from build123d import *

# Parameters (mm, degrees)
SKETCH1_W           = 70
SKETCH1_H           = 160
BOSS_EXTRUDE1_DEPTH = 6.35
SKETCH7_W           = 4.699
SKETCH7_H           = 2.5
FILLET1_R           = 18
SKETCH11_R          = 1.65
CUT_EXTRUDE4_DEPTH  = 3.5
SKETCH14_R          = 1.25
CUT_EXTRUDE7_DEPTH  = 3.5


with BuildPart() as part:
    # Sketch1 → Boss-Extrude1 (new body)
    with BuildSketch(Plane(origin=(0, 0, 0), x_dir=(1, 0, 0), z_dir=(0, 1, 0))):
        Rectangle(SKETCH1_W, SKETCH1_H)
    extrude(amount=BOSS_EXTRUDE1_DEPTH)

    # Cut-Sweep2: sweep along a path in Sketch2
    with BuildLine(Plane(origin=(0, 0, 0), x_dir=(1, 0, 0), z_dir=(0, 1, 0))) as cut_sweep2_path:
        Line((-13, 73), (13, 73))
        ThreePointArc((13, 73), (23.606601718, 68.606601718), (28, 58))
        Line((28, 58), (28, -58))
        ThreePointArc((28, -58), (23.606601718, -68.606601718), (13, -73))
        Line((13, -73), (-13, -73))
        ThreePointArc((-13, -73), (-23.606601718, -68.606601718), (-28, -58))
        Line((-28, -58), (-28, 58))
        ThreePointArc((-28, 58), (-23.606601718, 68.606601718), (-13, 73))
    # Sketch7 → Cut-Sweep2 (sweep, cut)
    with BuildSketch(Plane.XY):
        with Locations((28, 1.25)):
            Rectangle(SKETCH7_W, SKETCH7_H)
    sweep(path=cut_sweep2_path.line, mode=Mode.SUBTRACT)

    # Fillet1
    fillet1_edges = [part.edges().sort_by_distance(p)[0] for p in [
        (35, 3.175, 80),
        (-35, 3.175, 80),
        (-35, 3.175, -80),
        (35, 3.175, -80),
    ]]
    fillet(fillet1_edges, radius=FILLET1_R)

    # Sketch11 → Cut-Extrude4 (cut)
    with BuildSketch(Plane.XZ):
        with Locations(Location((16.535533906, 61.535533906, 0), (0, 0, 90))):
            Circle(SKETCH11_R)
        with Locations(Location((18, -20.511844635, 0), (0, 0, 270))):
            Circle(SKETCH11_R)
        with Locations(Location((18, 20.511844635, 0), (0, 0, 270))):
            Circle(SKETCH11_R)
        with Locations(Location((-16.535533906, 61.535533906, 0), (0, 0, 270))):
            Circle(SKETCH11_R)
        with Locations(Location((-18, 20.511844635, 0), (0, 0, 90))):
            Circle(SKETCH11_R)
        with Locations(Location((16.535533906, -61.535533906, 0), (0, 0, 270))):
            Circle(SKETCH11_R)
        with Locations(Location((-18, -20.511844635, 0), (0, 0, 90))):
            Circle(SKETCH11_R)
        with Locations(Location((-16.535533906, -61.535533906, 0), (0, 0, 90))):
            Circle(SKETCH11_R)
    extrude(amount=-CUT_EXTRUDE4_DEPTH, mode=Mode.SUBTRACT)

    # Sketch14 → Cut-Extrude7 (cut)
    with BuildSketch(Plane(origin=(0, 6.35, 0), x_dir=(1, 0, 0), z_dir=(0, 1, 0))):
        with Locations(Location((-16.51, -40.888057962, 0), (0, 0, 270))):
            Circle(SKETCH14_R)
        with Locations(Location((0, -40.888057962, 0), (0, 0, 270))):
            Circle(SKETCH14_R)
        with Locations(Location((16.51, -40.888057962, 0), (0, 0, 270))):
            Circle(SKETCH14_R)
        with Locations(Location((16.51, -73.146057962, 0), (0, 0, 270))):
            Circle(SKETCH14_R)
        with Locations(Location((0, -73.146057962, 0), (0, 0, 270))):
            Circle(SKETCH14_R)
        with Locations(Location((-16.51, -73.146057962, 0), (0, 0, 270))):
            Circle(SKETCH14_R)
        with Locations(Location((-25, -32.987253412, 0), (0, 0, 270))):
            Circle(SKETCH14_R)
        with Locations(Location((25, -32.987253412, 0), (0, 0, 270))):
            Circle(SKETCH14_R)
        with Locations(Location((25, 69.012746588, 0), (0, 0, 270))):
            Circle(SKETCH14_R)
        with Locations(Location((-25, 69.012746588, 0), (0, 0, 270))):
            Circle(SKETCH14_R)
    extrude(amount=-CUT_EXTRUDE7_DEPTH, mode=Mode.SUBTRACT)


solid = part.part
The listing builds one solid part. Answer for the finished solid, in the listing's coordinates (mm). A direction names the side the tool comes from. Coordinates: 2 decimals unless noted, no trailing zeros. Loops run counter-clockwise (first coordinate to the right, second up) from the corner with the lowest first, then second, coordinate; pieces in that order, holes last. Notation, with made-up numbers: (42, -13.75) -> (88, -13.75) arc R28 ccw to (88, 16.25) -> close; hole circle Ø3 at (4, 9.5). An arc over 180 degrees is marked (long way). Write item = value, one per line. Start each with the question number.
1) A cutting plane is placed at B-B (z = 46.5). Give the vertices of the cut face in (x, y), then the cut area to 3 significant figures.
2) A cutting plane is placed at A-A (x = -11). Give the vertices of the cut face in (y, z), then the cut area to 3 significant figures.
3) Straight lines are drawn through the part: line 1 (X direction, y = 1.5, z = -48.5); line 2 (X direction, y = 1.25, z = 62); line 3 (Z direction, x = -17, y = 4.25). For each, find the intervals that lie inside material, in ascending order. Write a range as from..to.
4) A cutting plane is placed at C-C (x = 28). Give the vertices of the cut face in (y, z), then the cut area to 3 significant figures.
5) A tool of negligible diameter and unlimited length cuts with its end or side. For faces 1 (the face through (29.587, 3.219, 74.867)), 2 (the face through (22.04, 1.23, 66.85)), from which of +Z, -Z, +X, -X, +Y, -Y can it reach the whole face along a straight path? Write none if from no direction.
6) Given pin 1 Ø1 at (y, z) = (3.5, -63) entering from -X; pin 2 Ø2 at (x, y) = (-20, 1.5) entering from -Z; pin 3 Ø2.5 at (x, z) = (18, -20.51) entering from -Y, each flat-ended and moving along its own axis, determine where each tip first touches the part or whether it passes through.
7) The mould has two halves that part along X. Classify faces 3 (the face through (0, 3, 80)), 4 (the face through (29.587, 3.219, -74.867)), 5 (the face through (-17.167, 1.726, 60.011)): released by +X, released by -X, zero draft, split by the parting line, or undercut.
Responses:
q1.outline = (-35, 0) -> (-30.35, 0) -> (-30.35, 2.5) -> (-25.65, 2.5) -> (-25.65, 0) -> (25.65, 0) -> (25.65, 2.5) -> (30.35, 2.5) -> (30.35, 0) -> (35, 0) -> (35, 6.35) -> (-35, 6.35) -> close
q1.area = 421 mm²
q2.outline = (0, -80) -> (6.35, -80) -> (6.35, 80) -> (0, 80) -> (0, 75.35) -> (2.5, 75.35) -> (2.5, 70.65) -> (0, 70.65) -> (0, -70.65) -> (2.5, -70.65) -> (2.5, -75.35) -> (0, -75.35) -> close
q2.area = 993 mm²
q3.line_1 = -35..-30.35, -25.65..25.65, 30.35..35
q3.line_2 = -35..-29.88, -25..-18.12, -14.95..14.95, 18.12..25, 29.88..35
q3.line_3 = -80..39.74, 42.04..72, 74.3..80
q4.outline = (0, -76.25) -> (6.35, -76.25) -> (6.35, 76.25) -> (0, 76.25) -> (0, 66.72) -> (2.5, 66.72) -> (2.5, -66.72) -> (0, -66.72) -> close
q4.area = 635 mm²
q5.face_1 = +Z, +X, +Y, -Y
q5.face_2 = -Y
q6.pin_1 = -34.99
q6.pin_2 = -79.89
q6.pin_3 = 3.5
q7.face_3 = zero draft
q7.face_4 = released by +X
q7.face_5 = undercut
